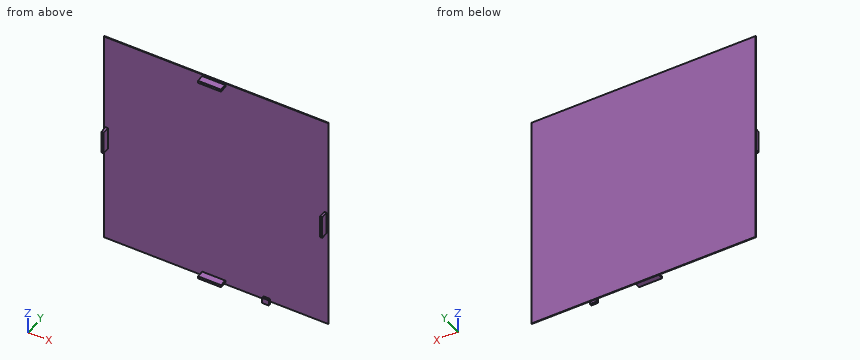
from build123d import *

# Parameters (mm, degrees)
SKETCH_W     = 495.3
SKETCH_H     = 495.3
PAD_DEPTH    = 1.5875
BOX_W        = 5.08
BOX_H        = 50.8
BOX_DEPTH    = 15.875
BOX001_W     = 5.08
BOX001_H     = 50.8
BOX001_DEPTH = 15.875
BOX002_W     = 50.8
BOX002_H     = 5.08
BOX002_DEPTH = 15.875
BOX003_W     = 50.8
BOX003_H     = 5.08
BOX003_DEPTH = 15.875
BOX004_W     = 15.24
BOX004_H     = 12.7
BOX004_DEPTH = 5.08


with BuildPart() as part:
    # Sketch → Pad (new body)
    with BuildSketch(Plane.XZ):
        with Locations((247.65, 247.65)):
            Rectangle(SKETCH_W, SKETCH_H)
    extrude(amount=PAD_DEPTH)

    # Box → Box (join)
    with BuildSketch(Plane(origin=(3.81, -1.5875, 222.25), x_dir=(1, 0, 0), z_dir=(0, -1, 0))):
        with Locations((2.54, 25.4)):
            Rectangle(BOX_W, BOX_H)
    extrude(amount=BOX_DEPTH)

    # Box001 → Box001 (join)
    with BuildSketch(Plane(origin=(486.41, -1.5875, 222.25), x_dir=(1, 0, 0), z_dir=(0, -1, 0))):
        with Locations((2.54, 25.4)):
            Rectangle(BOX001_W, BOX001_H)
    extrude(amount=BOX001_DEPTH)

    # Box002 → Box002 (join)
    with BuildSketch(Plane(origin=(217.17, -1.5875, 3.81), x_dir=(1, 0, 0), z_dir=(0, -1, 0))):
        with Locations((25.4, 2.54)):
            Rectangle(BOX002_W, BOX002_H)
    extrude(amount=BOX002_DEPTH)

    # Box003 → Box003 (join)
    with BuildSketch(Plane(origin=(217.17, -1.5875, 486.41), x_dir=(1, 0, 0), z_dir=(0, -1, 0))):
        with Locations((25.4, 2.54)):
            Rectangle(BOX003_W, BOX003_H)
    extrude(amount=BOX003_DEPTH)

    # Box004 → Box004 (join)
    with BuildSketch(Plane(origin=(351.79, -1.5875, -6.35), x_dir=(1, 0, 0), z_dir=(0, -1, 0))):
        with Locations((7.62, 6.35)):
            Rectangle(BOX004_W, BOX004_H)
    extrude(amount=BOX004_DEPTH)


solid = part.part
Can you work these out from the model? Positions are in its coordinate system, mm. Coordinates: 2 decimals unless noted, no trailing zeros. Write each loop counter-clockwise with the first axis right and the second up, starting at its lowest first coordinate (ties: lowest second). Pieces come first, ordered by that corner, then holes. Notation, with made-up numbers: (84, -39.5) - (131, -39.5) arc R28 ccw to (131, -12.5) - close; hole circle Ø5 at (5.25, -16.5). An arc over 180 degrees is marked (long way). Return JSON: item names as keys, results as strings. Group by question number.
Item 1: I'm going to push flat-ended pins straight in: pin 1 Ø2 at (x, z) = (330, 284) entering from -Y; pin 2 Ø5.5 at (y, z) = (-12.5, 489) entering from +X; pin 3 Ø5 at (x, y) = (231.5, -11.5) entering from +Z; pin 4 Ø8 at (y, z) = (-7.5, 347.5) entering from -X. Where does each tip first touch, or does it pass through?
Item 2: If we section it at D-D (z = 90): Write out the boundary of the cut face in (x, y), then the cut area to 3 significant figures.
Item 3: Please list where these lines run through material, in increasing order: probe 1 along Z at (x, y) = (241.5, -1.75); probe 2 along Y at (x, z) = (169, 370.5).
Item 4: If we section it at C-C (x = 43): Write out the boundary of the cut face in (y, z), then the cut area to 3 significant figures.
Item 5: If we section it at B-B (z = 255): Write out the boundary of the cut face in (x, y).
Item 6: If we section it at A-A (y = -14.25): Write out the boundary of the cut face in (x, z).
Return value:
{
 "1": {"pin 1": "stops at y = -1.59", "pin 2": "stops at x = 267.97", "pin 3": "stops at z = 491.49", "pin 4": "passes through"},
 "2": {"outline": "(0, -1.59) - (495.3, -1.59) - (495.3, 0) - (0, 0) - close", "area": "786 mm^2"},
 "3": {"probe 1": "z = 3.81 to 8.89, 486.41 to 491.49", "probe 2": "y = -1.59 to 0"},
 "4": {"outline": "(-1.59, 0) - (0, 0) - (0, 495.3) - (-1.59, 495.3) - close", "area": "786 mm^2"},
 "5": {"outline": "(0, -1.59) - (3.81, -1.59) - (3.81, -17.46) - (8.89, -17.46) - (8.89, -1.59) - (486.41, -1.59) - (486.41, -17.46) - (491.49, -17.46) - (491.49, -1.59) - (495.3, -1.59) - (495.3, 0) - (0, 0) - close"},
 "6": {"outline": "(3.81, 222.25) - (8.89, 222.25) - (8.89, 273.05) - (3.81, 273.05) - close; (217.17, 3.81) - (267.97, 3.81) - (267.97, 8.89) - (217.17, 8.89) - close; (217.17, 486.41) - (267.97, 486.41) - (267.97, 491.49) - (217.17, 491.49) - close; (486.41, 222.25) - (491.49, 222.25) - (491.49, 273.05) - (486.41, 273.05) - close"}
}
